Input: part model. Units: mm. Frame: model coordinates. Face numbers are marked on the shaded views. A direction names the side the tool comes from. Give positions to 0.01 mm unless a question says otherwise; leave off trailing zeros. Loops run counter-clockwise (first coordinate to the right, second up) from the corner with the lowest first, then second, coordinate; pieces in that order, holes last. Notation, with made-up numbers: M 46,47 L 104,47 A21 cw 104,51 Z; hole C -0.75,57.5 d8. An arc over 180 degrees is marked long. Use CSV: the item, a comma, the result in double quotes. Start each with the question number.
Q1. Section A-A, the plane y = 20. Output: boundary loops of the cut face in (x, z).
Q2. Section C-C, the plane y = 59. Output: boundary loops of the cut face in (x, z).
Q3. Section D-D, the plane z = -1.5. Output: boundary loops of the cut face in (x, y), plus the area to 3 significant figures.
Q4. Material intervals for line 1 along Y through (x, z) = (-21, -1.5); line 2 along X through (y, z) = (52.5, -1.5); line 3 along Z through (x, y) = (-17, 73.5), sorted ascending.
Q5. Section B-B, the plane x = -1.5. Output: boundary loops of the cut face in (y, z).
Q6. Pin query (flat end, axial travel): pin 1 (20 mm diameter, centred on y = 44.5, z = 3, fed in from +X); pin 2 (1.2 mm diameter, centred on x = -9.5, z = -21.5, fed in from -Y); pin 3 (18 mm diameter, centred on x = -8, y = 54.5, fed in from +Z). Return the tip coordinate at first contact, or that it passes through.
Q7. Reachability of the marked faces 1 and 2 from +Z, -Z, +X, -X, +Y, -Y: full face, straight path, thin tool, end or side. Return the list, or none.
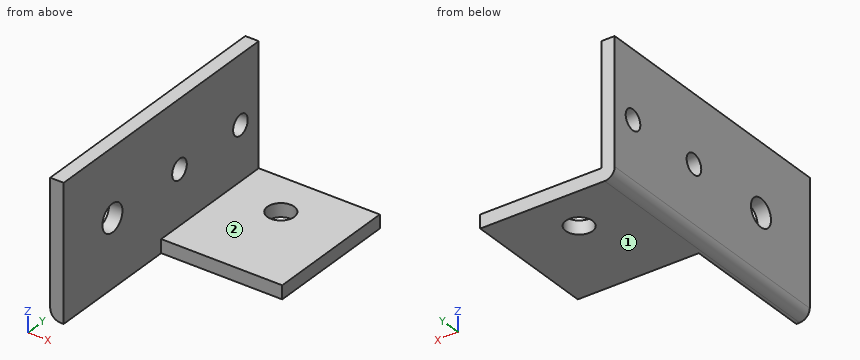
from build123d import *

# Parameters (mm, degrees)
EXTRUDE_THIN1_DEPTH   = 80
SKETCH5_R             = 4.1
SKETCH5_R_2           = 3
CUT_EXTRUDE2_DEPTH    = 10
SKETCH6_W             = 57.412547925
SKETCH6_H             = 40
CUT_EXTRUDE3_DEPTH    = 10
F_8_0MM_DOWEL_HOLE1_D = 8


with BuildPart() as part:
    # Sketch1 → Extrude-Thin1 (new body)
    with BuildSketch(Plane(origin=(0, 0, 0), x_dir=(1, 0, 0), z_dir=(0, 1, 0))):
        with BuildLine():
            Line((-22.658959538, -16.878612717), (-22.658959538, 20.121387283))
            ThreePointArc((-22.658959538, 20.121387283), (-21.780279881, 22.242707627), (-19.658959538, 23.121387283))
            Line((-19.658959538, 23.121387283), (17.341040462, 23.121387283))
            Line((17.341040462, 23.121387283), (17.341040462, 19.121387283))
            Line((17.341040462, 19.121387283), (-18.658959538, 19.121387283))
            Line((-18.658959538, 19.121387283), (-18.658959538, -16.878612717))
            Line((-18.658959538, -16.878612717), (-22.658959538, -16.878612717))
        make_face()
    extrude(amount=EXTRUDE_THIN1_DEPTH)

    # Sketch5 → Cut-Extrude2 (cut)
    with BuildSketch(Plane.ZY.offset(22.658959538)):
        with Locations((-3.121387283, 20)):
            Circle(SKETCH5_R)
        with Locations((-3.121387283, 47.5)):
            Circle(SKETCH5_R_2)
        with Locations((-3.121387283, 72.5)):
            Circle(SKETCH5_R_2)
    extrude(amount=-CUT_EXTRUDE2_DEPTH, mode=Mode.SUBTRACT)

    # Sketch6 → Cut-Extrude3 (cut)
    with BuildSketch(Plane(origin=(0, 0, -23.121387283), x_dir=(-1, 0, 0), z_dir=(0, 0, -1))):
        with Locations((-10.047314424, 20)):
            Rectangle(SKETCH6_W, SKETCH6_H)
    extrude(amount=-CUT_EXTRUDE3_DEPTH, mode=Mode.SUBTRACT)

    # Ø8.0mm Dowel Hole1 (through all)
    with Locations(Plane(origin=(0, 0, -23.121387283), x_dir=(-1, 0, 0), z_dir=(0, 0, -1))):
        with Locations((2.658959538, 67)):
            Hole(F_8_0MM_DOWEL_HOLE1_D / 2)


solid = part.part
A:
1,outline,"M -22.66,-20.12 A3 ccw -19.66,-23.12 L -18.66,-23.12 L -18.66,-7.22 L -22.66,-7.22 Z; M -22.66,0.98 L -18.66,0.98 L -18.66,16.88 L -22.66,16.88 Z"
2,outline,"M -22.66,-20.12 A3 ccw -19.66,-23.12 L 17.34,-23.12 L 17.34,-19.12 L -18.66,-19.12 L -18.66,16.88 L -22.66,16.88 Z"
3,outline,"M -22.66,0 L -18.66,0 L -18.66,16.23 L -22.66,16.23 Z; M -22.66,23.77 L -18.66,23.77 L -18.66,44.98 L -22.66,44.98 Z; M -22.66,50.02 L -18.66,50.02 L -18.66,69.98 L -22.66,69.98 Z; M -22.66,75.02 L -18.66,75.02 L -18.66,80 L -22.66,80 Z"
3,area,"249 mm^2"
4,line 1,"0 to 16.23, 23.77 to 44.98, 50.02 to 69.98, 75.02 to 80"
4,line 2,"-22.66 to -18.66"
4,line 3,"-23.12 to -19.12"
5,outline,"M 40,-23.12 L 63.17,-23.12 L 63.17,-19.12 L 40,-19.12 Z; M 70.83,-23.12 L 80,-23.12 L 80,-19.12 L 70.83,-19.12 Z"
6,pin 1,"x = -18.66"
6,pin 2,"y = 40"
6,pin 3,"z = -19.12"
7,face 1,"-Z, +X, -X, +Y, -Y"
7,face 2,"+Z, +X, +Y, -Y"
